```python
from build123d import *

# Parameters (mm, degrees)
F1_DEPTH = 400
F3_DEPTH = 290.001


# Not quite as in the source:
# - a feature names something its author has since deleted; it is built from what else it names


with BuildPart() as f1:
    # F0 (on Right) → F1 (new body)
    with BuildSketch(Plane.YZ):
        Polygon((-80, 0), (0, 0), (0, 501), (-1, 501), (-1, 1), (-79.5336923418, 1), (-289, 250.6322246791), (-289, 501), (-290, 501), (-290, 250.2682544448), align=None)
    extrude(amount=-F1_DEPTH)

    # F2 (on face) → F3 (cut, through all)
    with BuildSketch(Plane(origin=(0, 0, 0), x_dir=(-1, 0, 0), z_dir=(0, 1, 0))):
        Polygon((400, 0), (400, 240), (250, 80), (250, 0), align=None)
        Polygon((0, 0), (150, 0), (150, 80), (0, 240), align=None)
    extrude(amount=-F3_DEPTH, mode=Mode.SUBTRACT)


solid = f1.part
```
Read the model definition and answer for the solid it produces. Units are mm, in the model's axes. A direction names the side the tool comes from. Give positions to 0.01 mm unless a question says otherwise; leave off trailing zeros. Order: outer loops, then holes, each group sorted by start corner. A loop starts at its lowest first (then second) coordinate and runs counter-clockwise, first axis right, second up. Notation, with made-up numbers: (-24, 76) -> (24, 76) arc R17 cw to (24, 95) -> close; hole circle Ø3 at (76.5, -25.75). An arc over 180 degrees is marked (long way). Write item = value, one per line.
1. The mould has two halves that part along Y. Classify faces 3 (the face through (-76.05, -0.49, 158.88)), 4 (the face through (-197, 0, 303)), 5 (the face through (-199, -40, 1)): +Y half, -Y half, draft (parallel to the pull), parting line (faces both ways), or undercut.
Numbers:
face_3 = draft
face_4 = +Y half
face_5 = undercut
2. For faces 1 (the face through (-197.2, -206.075, 151.806)), 2 (the face through (-364.239, -248.432, 201.855)), determine the directions among +Z, -Z, +X, -X, +Y, -Y from which every point of the face is accessible in a straight line to the end or side of a thin tool.
Numbers:
face_1 = +Z, +X, -X
face_2 = -Z, -X, +Y, -Y
3. A cutting plane is placed at B-B, the plane x = -186. Write down the section's boundary in (y, z).
Numbers:
outline = (-290, 250.27) -> (-80, 0) -> (0, 0) -> (0, 501) -> (-1, 501) -> (-1, 1) -> (-79.53, 1) -> (-289, 250.63) -> (-289, 501) -> (-290, 501) -> close
4. A cutting plane is placed at D-D, the plane z = 219. Write down the section's boundary in (x, y), and give its area (3 significant figures).
Numbers:
outline = (-380.31, -263.76) -> (-19.69, -263.76) -> (-19.69, -262.46) -> (-380.31, -262.46) -> close; (-380.31, -1) -> (-19.69, -1) -> (-19.69, 0) -> (-380.31, 0) -> close
area = 831 mm²
5. A cutting plane is placed at C-C, the plane x = -341. Write down the section's boundary in (y, z), and give its area (3 significant figures).
Numbers:
outline = (-290, 250.27) -> (-228.58, 177.07) -> (-227.27, 177.07) -> (-289, 250.63) -> (-289, 501) -> (-290, 501) -> close; (-1, 177.07) -> (0, 177.07) -> (0, 501) -> (-1, 501) -> close
area = 670 mm²
6. Straight lines are drawn through the part: line 1 along Y through (x, z) = (-79.5, 261); line 2 along Y through (x, z) = (-181, 166); line 3 along Z through (x, y) = (-225, -68.5). For each, find the intervals that lie inside material, in ascending order.
Numbers:
line_1 = -290 to -289, -1 to 0
line_2 = -219.29 to -217.99, -1 to 0
line_3 = 0 to 1
7. Given pin 1 (2 mm diameter, centred on x = -102.5, y = -255, fed in from +Z), flat-ended and moving along its own axis, determine where the tip first touches the part or whether it passes through.
Numbers:
pin_1 = 211.3
8. A cutting plane is placed at A-A, the plane z = 316. Write down the section's boundary in (x, y), and give its area (3 significant figures).
Numbers:
outline = (-400, -290) -> (0, -290) -> (0, -289) -> (-400, -289) -> close; (-400, -1) -> (0, -1) -> (0, 0) -> (-400, 0) -> close
area = 800 mm²
